from build123d import *

# Parameters (mm, degrees)
SKETCH1_R           = 2.05
BOSS_EXTRUDE1_DEPTH = 6.5


with BuildPart() as part:
    # Sketch1 → Boss-Extrude1 (new body)
    with BuildSketch(Plane(origin=(-14.5, 0, 0), x_dir=(0, 0, -1), z_dir=(1, 0, 0))):
        with BuildLine():
            ThreePointArc((-17.5, -136.5), (-23.5, -130.5), (-29.5, -136.5))
            Line((-29.5, -136.5), (-30, -181))
            ThreePointArc((-30, -181), (-27.287286528, -186.019337335), (-21.602084238, -186.5))
            Line((-21.602084238, -186.5), (-24, -186.5))
            ThreePointArc((-24, -186.5), (-29.5, -181), (-24, -175.5))
            Line((-24, -175.5), (-17.938202247, -175.5))
            Line((-17.938202247, -175.5), (-17.5, -136.5))
        make_face()
        with Locations((-23.5, -136.5)):
            Circle(SKETCH1_R, mode=Mode.SUBTRACT)
        with BuildLine():
            Line((-24, -186.5), (-21.602084238, -186.5))
            ThreePointArc((-21.602084238, -186.5), (-18.980662665, -184.287286528), (-18, -181))
            Line((-18, -181), (-17.938202247, -175.5))
            Line((-17.938202247, -175.5), (-24, -175.5))
            ThreePointArc((-24, -175.5), (-29.5, -181), (-24, -186.5))
        make_face()
        with Locations((-24, -181)):
            Circle(SKETCH1_R, mode=Mode.SUBTRACT)
    extrude(amount=BOSS_EXTRUDE1_DEPTH)


solid = part.part
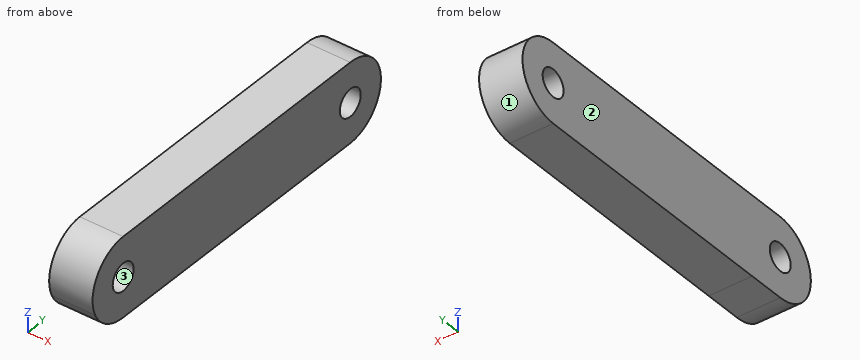
The model under review builds one solid part; all positions refer to its coordinate system, in mm. Face numbers are marked on the shaded views. Round coordinates to 2 decimals unless told otherwise and drop trailing zeros. Write each loop counter-clockwise with the first axis right and the second up, starting at its lowest first coordinate (ties: lowest second). Pieces come first, ordered by that corner, then holes. Notation, with made-up numbers: M 16,35 L 65,35 A24 ccw 65,71 Z; hole C 17.25,81.5 d8. An arc over 180 degrees is marked long. Use a Markdown table: item, result. Add a question column.
Q1. We need section A-A, the plane x = -8.5. State the section outline as (y, z) points, plus the area to 3 significant figures.
Q2. We need section D-D, the plane z = 29. State the section outline as (x, y) points, plus the area to 3 significant figures.
Q3. To check wall thickness, follow line 1 (Y direction, x = -13, z = 22.5); line 2 (Y direction, x = -11.75, z = 23.5); line 3 (Z direction, x = -12.25, y = -181). State the ranges of each line that lie inside material, in increasing order.
Q4. We need section C-C, the plane y = -146. State the section outline as (x, z) points, plus the area to 3 significant figures.
Q5. We need section B-B, the plane z = 24. State the section outline as (x, y) points.
Q6. Insertion check: pin 1 (1 mm diameter, centred on x = -11, z = 28, fed in from -Y); pin 2 (2 mm diameter, centred on x = -9.5, y = -171.5, fed in from -Z); pin 3 (3.5 mm diameter, centred on y = -136.5, z = 23.5, fed in from +X). Each pin has a flat end and moves straight along its axis. Give the tip position at first contact, or say it passes through.
Q7. The part is to be moulded in two halves that separate along Y. For the marked faces 1, 2 and 3, say which applies: pulls with the +Y half, pulls with the -Y half, needs draft (parallel to the pull), parting line crosses it, or undercut.
Findings below:
| question | item | result |
|---|---|---|
| 1 | outline | M -181,18 L -136.5,17.5 A6 ccw -136.5,29.5 L -181,30 A6 ccw Z; hole C -181,24 d4.1; hole C -136.5,23.5 d4.1 |
| 1 | area | 621 mm² |
| 2 | outline | M -14.5,-184.32 L -8,-184.32 L -8,-134.1 L -14.5,-134.1 Z |
| 2 | area | 326 mm² |
| 3 | line 1 | y = -186.81 to -182.4, -179.6 to -138.29, -134.71 to -130.58 |
| 3 | line 2 | y = -186.98 to -182.99, -179.01 to -138.55, -134.45 to -130.5 |
| 3 | line 3 | z = 18 to 21.95, 26.05 to 30 |
| 4 | outline | M -14.5,17.61 L -8,17.61 L -8,29.61 L -14.5,29.61 Z |
| 4 | area | 78.0 mm² |
| 5 | outline | M -14.5,-187 L -8,-187 L -8,-183.05 L -14.5,-183.05 Z; M -14.5,-178.95 L -8,-178.95 L -8,-138.49 L -14.5,-138.49 Z; M -14.5,-134.51 L -8,-134.51 L -8,-130.52 L -14.5,-130.52 Z |
| 6 | pin 1 | stops at y = -185.87 |
| 6 | pin 2 | stops at z = 17.88 |
| 6 | pin 3 | passes through |
| 7 | face 1 | pulls with the +Y half |
| 7 | face 2 | needs draft |
| 7 | face 3 | undercut |
